from build123d import *

# Parameters (mm, degrees)
BASE_FLANGE1_DEPTH            = 550
CUT_EXTRUDE1_REACH            = 588.109
EDGE_FLANGE1_STRIP_W          = 9.4732
EDGE_FLANGE1_STRIP_H          = 2
EDGE_FLANGE1_STRIP_CUT_DEPTH  = 430
EDGE_FLANGE1_RELIEF_W         = 10.4732
EDGE_FLANGE1_RELIEF_H         = 1
EDGE_FLANGE1_RELIEF_CUT_DEPTH = 2
EDGE_FLANGE1_DEPTH            = 430


# Sheet-metal steps are written as plain solids
with BuildPart() as part:
    # Sketch1 → Base-Flange1 (new body)
    with BuildSketch(Plane.XY):
        with BuildLine():
            Line((0, 0), (29.2634, 0))
            ThreePointArc((29.2634, 0), (29.784254855, 0.215745145), (30, 0.7366))
            Line((30, 0.7366), (30, 200))
            Line((30, 200), (32, 200))
            Line((32, 200), (32, 0.7366))
            ThreePointArc((32, 0.7366), (31.198468417, -1.198468417), (29.2634, -2))
            Line((29.2634, -2), (0, -2))
            Line((0, -2), (0, 0))
        make_face()
    extrude(amount=BASE_FLANGE1_DEPTH)

    # Sketch6 → Cut-Extrude1 (cut, up to next)
    with BuildSketch(Plane(origin=(32, 0, 0), x_dir=(0, 0, -1), z_dir=(1, 0, 0)), mode=Mode.PRIVATE) as cut_extrude1_sk1:
        Polygon((-550, 0.7366), (-430, 200), (-550, 200), align=None)
    cut_extrude1_tool1 = extrude(cut_extrude1_sk1.sketch, amount=-CUT_EXTRUDE1_REACH, mode=Mode.PRIVATE) & part.part
    add(cut_extrude1_tool1.solids().sort_by_distance((32, 133.578867, 510))[0], mode=Mode.SUBTRACT)

    # Edge-Flange1 strip (across the edge) → Edge-Flange1 strip cut (cut)
    with BuildSketch(Plane(origin=(32, 200, 0), x_dir=(0, -1, 0), z_dir=(0, 0, 1))):
        with Locations((-2, -1)):
            Rectangle(EDGE_FLANGE1_STRIP_W, EDGE_FLANGE1_STRIP_H)
    extrude(amount=EDGE_FLANGE1_STRIP_CUT_DEPTH, mode=Mode.SUBTRACT)

    # Edge-Flange1 relief (on the sheet) → Edge-Flange1 relief cut (cut)
    with BuildSketch(Plane(origin=(32, 197.2634, 0), x_dir=(0, -1, 0), z_dir=(1, 0, 0))):
        with Locations((-4.2366, -430.5)):
            Rectangle(EDGE_FLANGE1_RELIEF_W, EDGE_FLANGE1_RELIEF_H)
    extrude(amount=-EDGE_FLANGE1_RELIEF_CUT_DEPTH, mode=Mode.SUBTRACT)

    # Edge-Flange1 section (across the edge) → Edge-Flange1 (add)
    with BuildSketch(Plane(origin=(32, 200, 0), x_dir=(0, -1, 0), z_dir=(0, 0, 1))):
        with BuildLine():
            Line((0, 0.7366), (0, 38))
            Line((0, 38), (2, 38))
            Line((2, 38), (2, 0.7366))
            ThreePointArc((2, 0.7366), (2.215745145, 0.215745145), (2.7366, 0))
            Line((2.7366, 0), (2.7366, -2))
            ThreePointArc((2.7366, -2), (0.801531583, -1.198468417), (0, 0.7366))
        make_face()
    extrude(amount=EDGE_FLANGE1_DEPTH)


solid = part.part
Geometry: final body of the model. Coordinates: model frame, mm. A direction names the side the tool comes from. Give positions to 0.01 mm unless a question says otherwise; leave off trailing zeros. Loops run counter-clockwise (first coordinate to the right, second up) from the corner with the lowest first, then second, coordinate; pieces in that order, holes last. Notation, with made-up numbers: (-37.75, 61) - (13.25, 61) arc R27 cw to (13.25, 84) - close; hole circle Ø7 at (2.25, 29). An arc over 180 degrees is marked (long way). One line per question, with ' | ' between items. Start each with the question number.
(1) Section query C-C on y = 75. Return loops of the section in (x, z).
(2) Reachability of faces 1 (the flat face through (31.014, 98.155, 491.333)), 2 (the flat face through (52, 198, 212)), 3 (the flat face through (30, 98, 271)) from +Z, -Z, +X, -X, +Y, -Y: full face, straight path, thin tool, end or side. Return the list, or none.
(3) Ray query, line 1 (X direction, y = 105.5, z = 437.5); line 2 (Y direction, x = 9.5, z = 384); line 3 (Y direction, x = 48, z = 130). Return the intervals inside material, ascending. Write a range as from..to.
(4) Contact query for flat-ended pins moving along their axis: pin 1 (8 mm diameter, centred on y = 165.5, z = 287, fed in from -X); pin 2 (1 mm diameter, centred on x = 31, y = 197, fed in from -Z); pin 3 (12 mm diameter, centred on y = 143, z = 277, fed in from +X); pin 4 (1.1 mm diameter, centred on x = 56, y = 198.5, fed in from +Z). Output: stop coordinate, or through.
(5) Section query A-A on z = 103.5. Return loops of the section in (x, y).
(6) Section query B-B on x = 55. Return loops of the section in (y, z).
The answers:
1) outline: (30, 0) - (32, 0) - (32, 505.28) - (30, 505.28) - close
2) face 1: +Z, +X, -X, +Y | face 2: +Z, -Z, +X, -Y | face 3: +Z, -Z, -X, +Y
3) line 1: 30..32 | line 2: -2..0 | line 3: 198..200
4) pin 1: x = 30 | pin 2: z = 0 | pin 3: x = 32 | pin 4: z = 430
5) outline: (0, -2) - (29.26, -2) arc R2.74 ccw to (32, 0.74) - (32, 197.26) arc R0.74 cw to (32.74, 198) - (70, 198) - (70, 200) - (32.74, 200) arc R2.74 ccw to (30, 197.26) - (30, 0.74) arc R0.74 cw to (29.26, 0) - (0, 0) - close
6) outline: (198, 0) - (200, 0) - (200, 430) - (198, 430) - close
